from build123d import *

# Parameters (mm, degrees)
SKETCH_3_W           = 80
SKETCH_3_H           = 48
EXTRUDE_1_DEPTH      = 25
FILLET_1_R           = 2
SHELL_1_T            = 1.5
SKETCH_5_W           = 45
SKETCH_5_H           = 2
EXTRUDE_2_DEPTH      = 8
EXTRUDE_START        = 4.48
EXTRUDE_3_DEPTH      = 4.48
SKETCH_8_W           = 8
SKETCH_8_H           = 6
CUT_EXTRUDE_2_DEPTH  = 4.03
CUT_EXTRUDE_3_DEPTH  = 4.03
SKETCH_11_W          = 13
SKETCH_11_H          = 5
CUT_EXTRUDE_4_DEPTH  = 4.03
SKETCH_12_W          = 5
SKETCH_12_H          = 3
CUT_EXTRUDE_5_DEPTH  = 4.03
SKETCH_13_R          = 2.5
CUT_EXTRUDE_6_DEPTH  = 4.03
SKETCH_14_R          = 4
CUT_EXTRUDE_7_DEPTH  = 4.03
CUT_EXTRUDE_12_DEPTH = 4.03
SKETCH_16_W          = 10
SKETCH_16_H          = 5
CUT_EXTRUDE_13_DEPTH = 4.03


with BuildPart() as part:
    # Sketch 3 → Extrude 1 (new body)
    with BuildSketch(Plane(origin=(0, 0, 0), x_dir=(1, 0, 0), z_dir=(0, 1, 0))):
        Rectangle(SKETCH_3_W, SKETCH_3_H)
    extrude(amount=EXTRUDE_1_DEPTH)

    # Fillet 1
    fillet_1_edges = [part.edges().sort_by_distance(p)[0] for p in [
        (-40, 12.5, -24),
        (40, 12.5, -24),
        (40, 12.5, 24),
        (-40, 12.5, 24),
    ]]
    fillet(fillet_1_edges, radius=FILLET_1_R)

    # Shell 1 (no face opened: a closed hollow body)
    add(offset(amount=-SHELL_1_T, mode=Mode.PRIVATE), mode=Mode.SUBTRACT)

    # Sketch 5 → Extrude 2 (add)
    with BuildSketch(Plane(origin=(0, 0, 0), x_dir=(1, 0, 0), z_dir=(0, 1, 0))):
        with Locations((17.5, 0)):
            Rectangle(SKETCH_5_W, SKETCH_5_H)
    extrude(amount=EXTRUDE_2_DEPTH)

    # Sketch 7 → Extrude 3 (add)
    with BuildSketch(Plane(origin=(0, 0, 0), x_dir=(1, 0, 0), z_dir=(0, 1, 0)).offset(EXTRUDE_START)):
        with BuildLine():
            Line((40, -1), (-5, -1))
            Line((-5, -1), (-5, -24))
            Line((-5, -24), (38, -24))
            ThreePointArc((38, -24), (39.414213562, -23.414213562), (40, -22))
            Line((40, -22), (40, -1))
        make_face()
    extrude(amount=-EXTRUDE_3_DEPTH)

    # Sketch 8 → Cut-Extrude 2 (cut)
    with BuildSketch(Plane(origin=(40, 0, 0), x_dir=(0, 0, -1), z_dir=(1, 0, 0))):
        with Locations((12, 8.48)):
            Rectangle(SKETCH_8_W, SKETCH_8_H)
    extrude(amount=-CUT_EXTRUDE_2_DEPTH, mode=Mode.SUBTRACT)

    # Sketch 8_4 → Cut-Extrude 3 (cut)
    with BuildSketch(Plane(origin=(40, 0, 0), x_dir=(0, 0, -1), z_dir=(1, 0, 0))):
        with BuildLine():
            ThreePointArc((-7, 6.98), (-7.439339828, 5.919339828), (-8.5, 5.48))
            Line((-8.5, 5.48), (-15.5, 5.48))
            ThreePointArc((-15.5, 5.48), (-16.560660172, 5.919339828), (-17, 6.98))
            ThreePointArc((-17, 6.98), (-16.560660172, 8.040660172), (-15.5, 8.48))
            Line((-15.5, 8.48), (-8.5, 8.48))
            ThreePointArc((-8.5, 8.48), (-7.439339828, 8.040660172), (-7, 6.98))
        make_face()
    extrude(amount=-CUT_EXTRUDE_3_DEPTH, mode=Mode.SUBTRACT)

    # Sketch 11 → Cut-Extrude 4 (cut)
    with BuildSketch(Plane.ZY.offset(40)):
        with Locations((-11.5, 6.1)):
            Rectangle(SKETCH_11_W, SKETCH_11_H)
    extrude(amount=-CUT_EXTRUDE_4_DEPTH, mode=Mode.SUBTRACT)

    # Sketch 12 → Cut-Extrude 5 (cut)
    with BuildSketch(Plane(origin=(40, 0, 0), x_dir=(0, 0, -1), z_dir=(1, 0, 0))):
        with Locations((-1.5, 14.5)):
            Rectangle(SKETCH_12_W, SKETCH_12_H)
    extrude(amount=-CUT_EXTRUDE_5_DEPTH, mode=Mode.SUBTRACT)

    # Sketch 13 → Cut-Extrude 6 (cut)
    with BuildSketch(Plane(origin=(40, 0, 0), x_dir=(0, 0, -1), z_dir=(1, 0, 0))):
        with Locations((3, 21)):
            Circle(SKETCH_13_R)
        with Locations((-6, 21)):
            Circle(SKETCH_13_R)
    extrude(amount=-CUT_EXTRUDE_6_DEPTH, mode=Mode.SUBTRACT)

    # Sketch 14 → Cut-Extrude 7 (cut)
    with BuildSketch(Plane.ZY.offset(40)):
        with Locations((-11.5, 14.6)):
            Circle(SKETCH_14_R)
    extrude(amount=-CUT_EXTRUDE_7_DEPTH, mode=Mode.SUBTRACT)

    # Sketch 15 → Cut-Extrude 12 (cut)
    with BuildSketch(Plane(origin=(0, 25, 0), x_dir=(1, 0, 0), z_dir=(0, 1, 0))):
        with BuildLine():
            Line((38.5, -20.5), (38.5, 20.5))
            ThreePointArc((38.5, 20.5), (37.914213562, 21.914213562), (36.5, 22.5))
            Line((36.5, 22.5), (-36.5, 22.5))
            ThreePointArc((-36.5, 22.5), (-37.914213562, 21.914213562), (-38.5, 20.5))
            Line((-38.5, 20.5), (-38.5, -20.5))
            ThreePointArc((-38.5, -20.5), (-37.914213562, -21.914213562), (-36.5, -22.5))
            Line((-36.5, -22.5), (36.5, -22.5))
            ThreePointArc((36.5, -22.5), (37.914213562, -21.914213562), (38.5, -20.5))
        make_face()
    extrude(amount=-CUT_EXTRUDE_12_DEPTH, mode=Mode.SUBTRACT)

    # Sketch 16 → Cut-Extrude 13 (cut)
    with BuildSketch(Plane.ZY.offset(40)):
        with Locations((13, 7.98)):
            Rectangle(SKETCH_16_W, SKETCH_16_H)
    extrude(amount=-CUT_EXTRUDE_13_DEPTH, mode=Mode.SUBTRACT)


solid = part.part
Could you check a few things on this model? Use its own coordinates, in mm. A direction names the side the tool comes from. Give positions to 0.01 mm unless a question says otherwise; leave off trailing zeros. Write each loop counter-clockwise with the first axis right and the second up, starting at its lowest first coordinate (ties: lowest second). Pieces come first, ordered by that corner, then holes. Notation, with made-up numbers: (52.25, 69.25) -> (105.25, 69.25) arc R22 ccw to (105.25, 81.25) -> close; hole circle Ø6 at (1, -1.5). An arc over 180 degrees is marked (long way). Write each question's results on one line, items separated by ' | '. Start each with the question number.
Q1. Suppose I cut it at D-D, the plane z = -11.5. List the corners of the cut face in (x, y) for me, and give its area (3 significant figures).
Q2. Suppose I cut it at A-A, the plane y = 21. List the corners of the cut face in (x, z) for me, and give its area (3 significant figures).
Q3. I need wall thicknesses on probe 1 along Z at (x, y) = (22.5, 7); probe 2 along Y at (x, z) = (-38.85, -11.5); probe 3 along Y at (x, z) = (39, 6). Which ranges of each line are inside material? Lowest first, please.
Q4. Suppose I cut it at C-C, the plane x = 29. List the corners of the cut face in (y, z) for me, and give its area (3 significant figures).
Q5. We'd pull the mould along Z, two halves only. Please class faces 1 (the face through (-12, 25, -23)), 2 (the face through (-39, 8.6, -12)), 3 (the face through (39.4, 12.68, 23.43)): +Z half, -Z half, draft (parallel to the pull), parting line (faces both ways), or undercut.
Q6. Suppose I cut it at B-B, the plane z = -3. List the corners of the cut face in (x, y) for me, and give its area (3 significant figures).
Q7. Which directions (+Z, -Z, +X, -X, +Y, -Y) give clear straight access to the entire face, cutting with the end or side of a thin tool? Please do faces 4 (the face through (39, 8, -8)), 5 (the face through (38, 23.5, -22.1)), 6 (the face through (-37.9, 24.26, -21.93)).
Q8. I'm going to push flat-ended pins straight in: pin 1 Ø5 at (x, z) = (-16, 8.5) entering from +Y; pin 2 Ø3 at (x, z) = (24, 18) entering from -Y; pin 3 Ø6.5 at (y, z) = (14.6, -11.5) entering from -X; pin 4 Ø1.2 at (x, y) = (-39.5, 8) entering from -Z. Where does each tip first touch, or does it pass through?
Outcome:
1) outline: (-40, 0) -> (40, 0) -> (40, 5.48) -> (38.5, 5.48) -> (38.5, 1.5) -> (-38.5, 1.5) -> (-38.5, 3.6) -> (-40, 3.6) -> close; (-40, 8.6) -> (-38.5, 8.6) -> (-38.5, 10.6) -> (-40, 10.6) -> close; (-40, 18.6) -> (-38.5, 18.6) -> (-38.5, 25) -> (-40, 25) -> close; (38.5, 11.48) -> (40, 11.48) -> (40, 25) -> (38.5, 25) -> close | area: 162 mm2
2) outline: (-40, -22) arc R2 ccw to (-38, -24) -> (38, -24) arc R2 ccw to (40, -22) -> (40, -5.5) -> (38.5, -5.5) -> (38.5, -22) arc R0.5 cw to (38, -22.5) -> (-38, -22.5) arc R0.5 cw to (-38.5, -22) -> (-38.5, 22) arc R0.5 cw to (-38, 22.5) -> (38, 22.5) arc R0.5 cw to (38.5, 22) -> (38.5, 8.5) -> (40, 8.5) -> (40, 22) arc R2 ccw to (38, 24) -> (-38, 24) arc R2 ccw to (-40, 22) -> close; (38.5, -0.5) -> (40, -0.5) -> (40, 3.5) -> (38.5, 3.5) -> close | area: 357 mm2
3) probe 1: -24 to -22.5, -1 to 1, 22.5 to 24 | probe 2: 0 to 3.6, 8.6 to 10.6, 18.6 to 25 | probe 3: 0 to 18.5, 23.5 to 25
4) outline: (0, -24) -> (25, -24) -> (25, -22.5) -> (1.5, -22.5) -> (1.5, -1) -> (8, -1) -> (8, 1) -> (4.48, 1) -> (4.48, 22.5) -> (25, 22.5) -> (25, 24) -> (0, 24) -> close | area: 220 mm2
5) face 1: draft | face 2: undercut | face 3: +Z half
6) outline: (-40, 0) -> (40, 0) -> (40, 18.5) -> (38.5, 18.5) -> (38.5, 1.5) -> (-38.5, 1.5) -> (-38.5, 25) -> (-40, 25) -> close; (38.5, 23.5) -> (40, 23.5) -> (40, 25) -> (38.5, 25) -> close | area: 183 mm2
7) face 4: +X | face 5: none | face 6: +Y
8) pin 1: y = 1.5 | pin 2: y = 0 | pin 3: x = 38.5 | pin 4: z = -23.79
